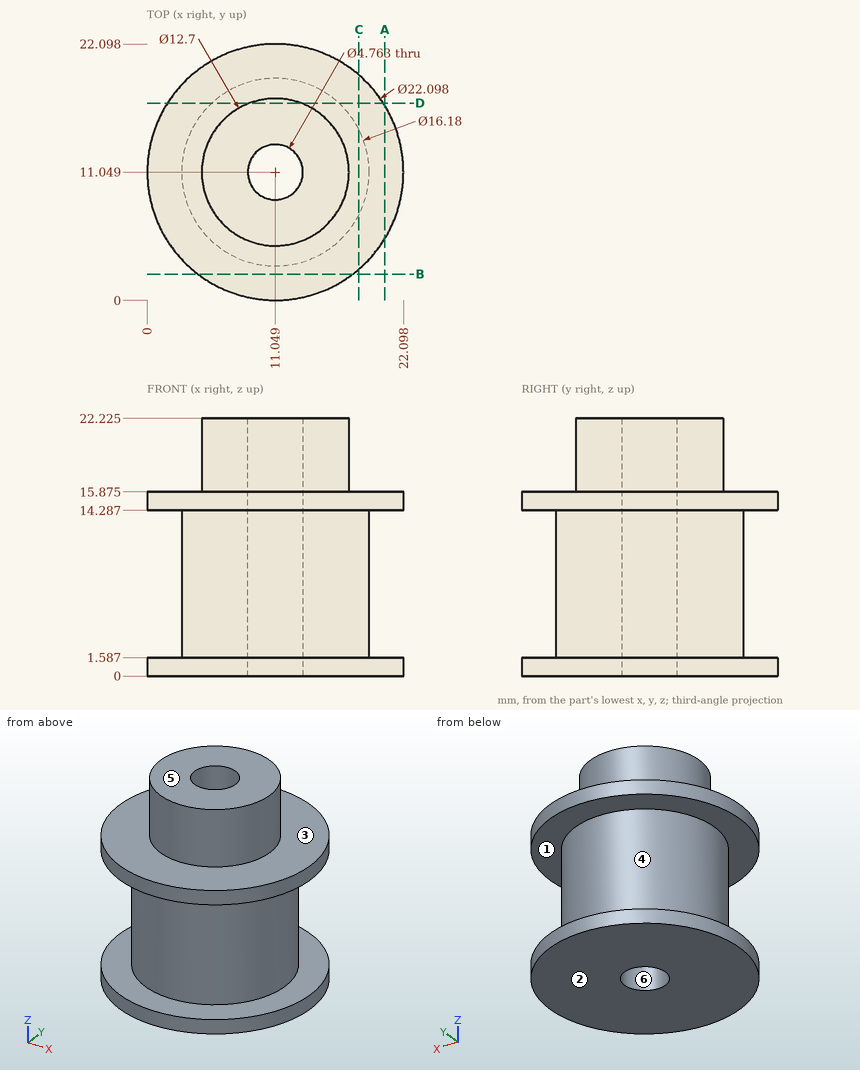
The drawing under review shows one solid part. Ordinate dimensions are in mm from its lowest x, y, z. A direction names the side the tool comes from. Coordinates: 2 decimals unless noted, no trailing zeros. Order: outer loops, then holes, each group sorted by start corner. A loop starts at its lowest first (then second) coordinate and runs counter-clockwise, first axis right, second up. Notation, with made-up numbers: (-36, -13.75) -> (5, -13.75) arc R16 ccw to (5, -3.75) -> close; hole circle Ø10 at (72, 28.5). An arc over 180 degrees is marked (long way). Use CSV: the item, a comma, the result in double quotes. Start each with the question number.
Item 1: For the marked faces 1, 2 and 3, list the 3-axis set-ups (+Z, -Z, +X, -X, +Y, -Y) from which the entire face can be reached by the end or side of a thin tool; tool diameter is ignored.
Item 2: We need section D-D, the plane y = 17. Give the boundary of the cut face in (x, z) (1 decimal).
Item 3: Wall thickness on probe 1 along Z at (x, y) = (6.5, 2.5) (1 decimal); probe 2 along Z at (x, y) = (15.75, 17.5) (1 decimal); probe 3 along X at (y, z) = (11.5, 4.5) (1 decimal): over which ranges is each line inside the solid? List them lowest first.
Item 4: Insertion check: pin 1 (5 mm diameter, centred on x = 13, z = 5, fed in from -Y); pin 2 (4.5 mm diameter, centred on x = 11.049, y = 11.049, fed in from -Z); pin 3 (5 mm diameter, centred on y = 18, z = 6.5, fed in from -X) (1 decimal); pin 4 (2 mm diameter, centred on x = 16.5, z = 11, fed in from -Y) (1 decimal). Each pin has a flat end and moves straight along its axis. Give the tip position at first contact, or say it passes through.
Item 5: We need section B-B, the plane y = 2.25. Give the boundary of the cut face in (x, z) (1 decimal).
Item 6: Draft analysis for pull direction Y (two halves, no side actions). For the marked faces 4, 5 and 6, state which applies: pulls with the +Y half, pulls with the -Y half, needs draft (parallel to the pull), parting line crosses it, or undercut.
Item 7: We need section A-A, the plane x = 20.5. Give the boundary of the cut face in (y, z) (1 decimal).
Item 8: We need section C-C, the plane x = 18.25. Give the boundary of the cut face in (y, z) (1 decimal).
Derived:
1,face 1,"none"
1,face 2,"-Z, +X, -X, +Y, -Y"
1,face 3,"+Z"
2,outline,"(1.7, 0) -> (20.4, 0) -> (20.4, 1.6) -> (16.5, 1.6) -> (16.5, 14.3) -> (20.4, 14.3) -> (20.4, 15.9) -> (13.3, 15.9) -> (13.3, 22.2) -> (8.8, 22.2) -> (8.8, 15.9) -> (1.7, 15.9) -> (1.7, 14.3) -> (5.6, 14.3) -> (5.6, 1.6) -> (1.7, 1.6) -> close"
3,probe 1,"z = 0 to 1.6, 14.3 to 15.9"
3,probe 2,"z = 0 to 15.9"
3,probe 3,"x = 3 to 8.7, 13.4 to 19.1"
4,pin 1,"stops at y = 2.96"
4,pin 2,"passes through"
4,pin 3,"stops at x = 4.3"
4,pin 4,"stops at y = 4.3"
5,outline,"(4.4, 0) -> (17.7, 0) -> (17.7, 1.6) -> (4.4, 1.6) -> close; (4.4, 14.3) -> (17.7, 14.3) -> (17.7, 15.9) -> (4.4, 15.9) -> close"
6,face 4,"parting line crosses it"
6,face 5,"needs draft"
6,face 6,"undercut"
7,outline,"(5.3, 0) -> (16.8, 0) -> (16.8, 1.6) -> (5.3, 1.6) -> close; (5.3, 14.3) -> (16.8, 14.3) -> (16.8, 15.9) -> (5.3, 15.9) -> close"
8,outline,"(2.7, 0) -> (19.4, 0) -> (19.4, 1.6) -> (14.7, 1.6) -> (14.7, 14.3) -> (19.4, 14.3) -> (19.4, 15.9) -> (2.7, 15.9) -> (2.7, 14.3) -> (7.4, 14.3) -> (7.4, 1.6) -> (2.7, 1.6) -> close"
